The listing builds one solid part. Answer for the finished solid, in the listing's coordinates (mm). Give positions to 0.01 mm unless a question says otherwise; leave off trailing zeros. Order: outer loops, then holes, each group sorted by start corner. A loop starts at its lowest first (then second) coordinate and runs counter-clockwise, first axis right, second up.
```python
from build123d import *

# Parameters (mm, degrees)
SKETCH1_W                                      = 50
SKETCH1_H                                      = 50
BOSS_EXTRUDE2_DEPTH                            = 4
BOSS_EXTRUDE3_START                            = 4
SKETCH1_4_R                                    = 2.5
BOSS_EXTRUDE3_DEPTH                            = 1
BOSS_EXTRUDE4_START                            = 4
SKETCH1_5_R                                    = 2.5
BOSS_EXTRUDE4_DEPTH                            = 3
CSK_FOR_M2_FLAT_HEAD_MACHINE_SCREW1_AT_2_COUNT = 2
CSK_FOR_M2_FLAT_HEAD_MACHINE_SCREW1_AT_2_PITCH = 8
CSK_FOR_M2_FLAT_HEAD_MACHINE_SCREW1_AT_3_COUNT = 2
CSK_FOR_M2_FLAT_HEAD_MACHINE_SCREW1_AT_3_PITCH = 16
CSK_FOR_M2_FLAT_HEAD_MACHINE_SCREW1_AT_4_COUNT = 2
CSK_FOR_M2_FLAT_HEAD_MACHINE_SCREW1_AT_4_PITCH = 24
CSK_FOR_M2_FLAT_HEAD_MACHINE_SCREW1_AT_5_COUNT = 2
CSK_FOR_M2_FLAT_HEAD_MACHINE_SCREW1_AT_5_PITCH = 32
CSK_FOR_M2_FLAT_HEAD_MACHINE_SCREW2_AT_2_COUNT = 2
CSK_FOR_M2_FLAT_HEAD_MACHINE_SCREW2_AT_2_PITCH = 32
CSK_FOR_M2_FLAT_HEAD_MACHINE_SCREW2_AT_3_COUNT = 2
CSK_FOR_M2_FLAT_HEAD_MACHINE_SCREW2_AT_3_PITCH = 24
CSK_FOR_M2_FLAT_HEAD_MACHINE_SCREW2_AT_4_COUNT = 2
CSK_FOR_M2_FLAT_HEAD_MACHINE_SCREW2_AT_4_PITCH = 16
CSK_FOR_M2_FLAT_HEAD_MACHINE_SCREW2_AT_5_COUNT = 2
CSK_FOR_M2_FLAT_HEAD_MACHINE_SCREW2_AT_5_PITCH = 8


with BuildPart() as part:
    # Sketch1 → Boss-Extrude2 (new body)
    with BuildSketch(Plane(origin=(0, 0, 0), x_dir=(1, 0, 0), z_dir=(0, 1, 0))):
        Rectangle(SKETCH1_W, SKETCH1_H)
    extrude(amount=BOSS_EXTRUDE2_DEPTH)

    # Sketch1<4> → Boss-Extrude3 (add)
    with BuildSketch(Plane(origin=(0, 0, 0), x_dir=(1, 0, 0), z_dir=(0, 1, 0)).offset(BOSS_EXTRUDE3_START)):
        with Locations(Location((-14.142135624, 14.142135624, 0), (0, 0, 90))):
            Circle(SKETCH1_4_R)
        with Locations(Location((-6.142135624, 14.142135624, 0), (0, 0, 90))):
            Circle(SKETCH1_4_R)
        with Locations(Location((9.857864376, 14.142135624, 0), (0, 0, 90))):
            Circle(SKETCH1_4_R)
        with Locations(Location((17.857864376, 14.142135624, 0), (0, 0, 90))):
            Circle(SKETCH1_4_R)
        with Locations(Location((1.857864376, 14.142135624, 0), (0, 0, 90))):
            Circle(SKETCH1_4_R)
    extrude(amount=BOSS_EXTRUDE3_DEPTH)

    # Sketch1<5> → Boss-Extrude4 (add)
    with BuildSketch(Plane(origin=(0, 0, 0), x_dir=(1, 0, 0), z_dir=(0, 1, 0)).offset(BOSS_EXTRUDE4_START)):
        with Locations(Location((14.142135624, -14.142135624, 0), (0, 0, 90))):
            Circle(SKETCH1_5_R)
        with Locations(Location((6.142135624, -14.142135624, 0), (0, 0, 90))):
            Circle(SKETCH1_5_R)
        with Locations(Location((-1.857864376, -14.142135624, 0), (0, 0, 90))):
            Circle(SKETCH1_5_R)
        with Locations(Location((-9.857864376, -14.142135624, 0), (0, 0, 90))):
            Circle(SKETCH1_5_R)
        with Locations(Location((-17.857864376, -14.142135624, 0), (0, 0, 90))):
            Circle(SKETCH1_5_R)
    extrude(amount=BOSS_EXTRUDE4_DEPTH)

    # Sketch3 → CSK for M2 Flat Head Machine Screw1 (revolve, cut)
    with BuildSketch(Plane(origin=(-14.142135624, 5, -14.142135624), x_dir=(0, 0, 1), z_dir=(1, 0, 0))):
        Polygon((0, 0), (0, 3.5), (1.5, 3.5), (1.5, 0.503826859), (1.635, 0), align=None)
    csk_for_m2_flat_head_machine_screw1 = revolve(axis=Axis((-14.142135624, 11.35, -14.142135624), (0, -1, 0)), mode=Mode.SUBTRACT)

    # CSK for M2 Flat Head Machine Screw1 at 2: CSK for M2 Flat Head Machine Screw1 ×2
    with Locations(*[(i * CSK_FOR_M2_FLAT_HEAD_MACHINE_SCREW1_AT_2_PITCH, 0, 0) for i in range(1, CSK_FOR_M2_FLAT_HEAD_MACHINE_SCREW1_AT_2_COUNT)]):
        add(csk_for_m2_flat_head_machine_screw1, mode=Mode.SUBTRACT)

    # CSK for M2 Flat Head Machine Screw1 at 3: CSK for M2 Flat Head Machine Screw1 ×2
    with Locations(*[(i * CSK_FOR_M2_FLAT_HEAD_MACHINE_SCREW1_AT_3_PITCH, 0, 0) for i in range(1, CSK_FOR_M2_FLAT_HEAD_MACHINE_SCREW1_AT_3_COUNT)]):
        add(csk_for_m2_flat_head_machine_screw1, mode=Mode.SUBTRACT)

    # CSK for M2 Flat Head Machine Screw1 at 4: CSK for M2 Flat Head Machine Screw1 ×2
    with Locations(*[(i * CSK_FOR_M2_FLAT_HEAD_MACHINE_SCREW1_AT_4_PITCH, 0, 0) for i in range(1, CSK_FOR_M2_FLAT_HEAD_MACHINE_SCREW1_AT_4_COUNT)]):
        add(csk_for_m2_flat_head_machine_screw1, mode=Mode.SUBTRACT)

    # CSK for M2 Flat Head Machine Screw1 at 5: CSK for M2 Flat Head Machine Screw1 ×2
    with Locations(*[(i * CSK_FOR_M2_FLAT_HEAD_MACHINE_SCREW1_AT_5_PITCH, 0, 0) for i in range(1, CSK_FOR_M2_FLAT_HEAD_MACHINE_SCREW1_AT_5_COUNT)]):
        add(csk_for_m2_flat_head_machine_screw1, mode=Mode.SUBTRACT)

    # Sketch5 → CSK for M2 Flat Head Machine Screw2 (revolve, cut)
    with BuildSketch(Plane(origin=(14.142135624, 7, 14.142135624), x_dir=(0, 0, 1), z_dir=(1, 0, 0))):
        Polygon((0, 0), (0, 6), (1.5, 6), (1.5, 0.503826859), (1.635, 0), align=None)
    csk_for_m2_flat_head_machine_screw2 = revolve(axis=Axis((14.142135624, 13.35, 14.142135624), (0, -1, 0)), mode=Mode.SUBTRACT)

    # CSK for M2 Flat Head Machine Screw2 at 2: CSK for M2 Flat Head Machine Screw2 ×2
    with Locations(*[(-i * CSK_FOR_M2_FLAT_HEAD_MACHINE_SCREW2_AT_2_PITCH, 0, 0) for i in range(1, CSK_FOR_M2_FLAT_HEAD_MACHINE_SCREW2_AT_2_COUNT)]):
        add(csk_for_m2_flat_head_machine_screw2, mode=Mode.SUBTRACT)

    # CSK for M2 Flat Head Machine Screw2 at 3: CSK for M2 Flat Head Machine Screw2 ×2
    with Locations(*[(-i * CSK_FOR_M2_FLAT_HEAD_MACHINE_SCREW2_AT_3_PITCH, 0, 0) for i in range(1, CSK_FOR_M2_FLAT_HEAD_MACHINE_SCREW2_AT_3_COUNT)]):
        add(csk_for_m2_flat_head_machine_screw2, mode=Mode.SUBTRACT)

    # CSK for M2 Flat Head Machine Screw2 at 4: CSK for M2 Flat Head Machine Screw2 ×2
    with Locations(*[(-i * CSK_FOR_M2_FLAT_HEAD_MACHINE_SCREW2_AT_4_PITCH, 0, 0) for i in range(1, CSK_FOR_M2_FLAT_HEAD_MACHINE_SCREW2_AT_4_COUNT)]):
        add(csk_for_m2_flat_head_machine_screw2, mode=Mode.SUBTRACT)

    # CSK for M2 Flat Head Machine Screw2 at 5: CSK for M2 Flat Head Machine Screw2 ×2
    with Locations(*[(-i * CSK_FOR_M2_FLAT_HEAD_MACHINE_SCREW2_AT_5_PITCH, 0, 0) for i in range(1, CSK_FOR_M2_FLAT_HEAD_MACHINE_SCREW2_AT_5_COUNT)]):
        add(csk_for_m2_flat_head_machine_screw2, mode=Mode.SUBTRACT)


solid = part.part
```
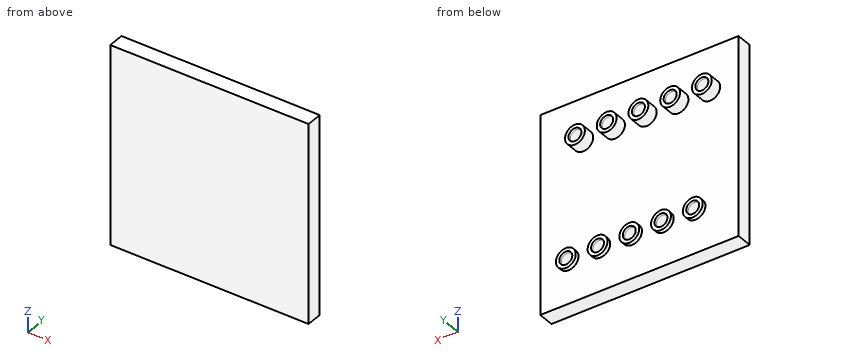
1) Find section A-A (y = 2.5). Count the separate pieces of the cut face and the enclosed holes in it, then the cut area to 3 significant figures.
Geometry says:
separate pieces: 1
enclosed holes: 10
area: 2,430 mm2
2) Straight lines are drawn through the part: probe 1 along Y at (x, z) = (4.5, -9); probe 2 along X at (y, z) = (4.75, 12.5); probe 3 along Z at (x, y) = (6, 2). For each, find the intervals that lie inside material, in ascending order.
Geometry says:
probe 1: y = 0 to 4
probe 2: x = -19.74 to -15.97, -11.74 to -7.97, -3.74 to 0.03, 4.26 to 8.03, 12.26 to 16.03
probe 3: z = -25 to 12.65, 15.64 to 25
3) Find section B-B (z = 5.5). Write down the section's boundary in (x, y), then the cut area to 3 significant figures.
Geometry says:
outline: (-25, 0) - (25, 0) - (25, 4) - (-25, 4) - close
area: 200 mm2
4) Given P1, Ø0.9, axis at x = -18, z = 14.5, coming from the +Y side; P2, Ø5.5, axis at x = 2, z = -14, coming from the +Y side; P3, Ø5, axis at x = 1.86, z = -14.14, coming from the -Y side; P4, Ø2, axis at x = 12, y = 5.5, coming from the -Z side, each flat-ended and moving along its own axis, determine where each tip first touches the part or whether it passes through.
Geometry says:
P1: stops at y = 1
P2: stops at y = 5
P3: stops at y = 0
P4: stops at z = -16.29
